```python
from build123d import *

# Parameters (mm, degrees)
SKETCH1_R                 = 10
BOSS_EXTRUDE1_DEPTH       = 25
FILLET2_R                 = 5
FILLET3_R                 = 5
F_3_0MM_DOWEL_HOLE1_D     = 3
F_3_0MM_DOWEL_HOLE1_DEPTH = 12.4
F_3_0MM_DOWEL_HOLE1_TIP   = 0.901290929


with BuildPart() as part:
    # Sketch1 → Boss-Extrude1 (new body)
    with BuildSketch(Plane(origin=(0, 0, 0), x_dir=(1, 0, 0), z_dir=(0, 1, 0))):
        with BuildLine():
            Line((0, 0), (-28, 0))
            Line((-28, 0), (-28, 8))
            Line((-28, 8), (-11.761010247, 8))
            ThreePointArc((-11.761010247, 8), (0, 32.310136302), (11.761010247, 8))
            Line((11.761010247, 8), (28, 8))
            Line((28, 8), (28, 0))
            Line((28, 0), (0, 0))
        make_face()
        with Locations(Location((0, 17.310136302, 0), (0, 0, 270))):
            Circle(SKETCH1_R, mode=Mode.SUBTRACT)
    extrude(amount=BOSS_EXTRUDE1_DEPTH)

    # Fillet2
    fillet2_edges = [part.edges().sort_by_distance(p)[0] for p in [
        (11.761010247, 12.5, -8),
    ]]
    fillet(fillet2_edges, radius=FILLET2_R)

    # Fillet3
    fillet3_edges = [part.edges().sort_by_distance(p)[0] for p in [
        (-11.761010247, 12.5, -8),
    ]]
    fillet(fillet3_edges, radius=FILLET3_R)

    # Ø3.0mm Dowel Hole1
    with Locations(Plane(origin=(23, 12.5, -8), x_dir=(-1, 0, 0), z_dir=(0, 0, -1))):
        with Locations((0, 0), (46.765023362, 0)):
            Hole(F_3_0MM_DOWEL_HOLE1_D / 2, depth=F_3_0MM_DOWEL_HOLE1_DEPTH)
            with Locations((0, 0, -(F_3_0MM_DOWEL_HOLE1_DEPTH + F_3_0MM_DOWEL_HOLE1_TIP / 2))):  # 118° drill point
                Cone(0, F_3_0MM_DOWEL_HOLE1_D / 2, F_3_0MM_DOWEL_HOLE1_TIP, mode=Mode.SUBTRACT)


solid = part.part
```
Geometry check sheet. Reference: the model listing, model coordinates, mm. A direction names the side the tool comes from. Give positions to 0.01 mm unless a question says otherwise; leave off trailing zeros. Order: outer loops, then holes, each group sorted by start corner. A loop starts at its lowest first (then second) coordinate and runs counter-clockwise, first axis right, second up. Notation, with made-up numbers: (1, 62) - (17, 62) arc R6 ccw to (17, 72) - close; hole circle Ø10 at (60, 85). An arc over 180 degrees is marked (long way). Answer in a Markdown table with one row per item. Add a question column.
Q1. Material ranges on probe 1 along Y at (x, z) = (23, -1); probe 2 along X at (y, z) = (4.25, -13.5); probe 3 along Z at (x, y) = (-24, 4.5), recorded low to high. Write a range as from..to.
Q2. Cross-section at A-A, the plane y = 12.5. Enter the section's corners in (x, z).
Q3. Gauge pin test, flat ends, axial feed: pin 1 (2.5 mm diameter, centred on x = -23.77, y = 12.5, fed in from +Z); pin 2 (8 mm diameter, centred on y = 5, z = -25, fed in from +X); pin 3 (4 mm diameter, centred on x = 23, y = 12.5, fed in from -Z); pin 4 (6 mm diameter, centred on y = 5.5, z = -20, fed in from +X). Record the tip position at first contact, or that the pin passes through.
Q4. Cross-section at B-B, the plane x = 23. Enter the section's corners in (y, z), then the cut area to 3 significant figures.
Q5. Mould release check, pull along X, two halves, no side actions. Record for faces 3 (the flat face through (25, 12, -8)), 4 (the flat face through (28, 12, -4)), 5 (the cylindrical face through (21.5, 12.57, -3.94)): pulls with the +X half, pulls with the -X half, needs draft (parallel to the pull), parting line crosses it, or undercut.
Q6. Cross-section at C-C, the plane z = -11.5. Enter the section's corners in (x, y), then the cut area to 3 significant figures.
Q7. Cross-section at D-D, the plane y = 4.5. Enter the section's corners in (x, z).
Q8. Tool access check on faces 1 (the flat face through (-22, 12, -8)), 2 (the flat face through (0, 0, -6)). Record the directions out of +Z, -Z, +X, -X, +Y, -Y that give a thin tool (end or side, any length) a straight path to the whole face; none if there is none.
Check values:
| question | item | result |
|---|---|---|
| 1 | probe 1 | y = 0..11, 14..25 |
| 1 | probe 2 | x = -14.56..-9.25, 9.25..14.56 |
| 1 | probe 3 | z = -8..0 |
| 2 | outline | (-28, -8) - (-25.27, -8) - (-25.27, 0) - (-28, 0) - close; (-22.27, -8) - (-19.53, -8) arc R5 cw to (-14.65, -14.08) arc R15 ccw (long way) to (14.65, -14.08) arc R5 cw to (19.53, -8) - (21.5, -8) - (21.5, 0) - (-22.27, 0) - close; (24.5, -8) - (28, -8) - (28, 0) - (24.5, 0) - close; hole circle Ø20 at (0, -17.31) |
| 3 | pin 1 | passes through |
| 3 | pin 2 | stops at x = 14.54 |
| 3 | pin 3 | stops at z = -8 |
| 3 | pin 4 | stops at x = 15 |
| 4 | outline | (0, -8) - (11, -8) - (11, 0) - (0, 0) - close; (14, -8) - (25, -8) - (25, 0) - (14, 0) - close |
| 4 | area | 176 mm^2 |
| 5 | face 3 | needs draft |
| 5 | face 4 | pulls with the +X half |
| 5 | face 5 | undercut |
| 6 | outline | (-14.76, 0) - (-8.14, 0) - (-8.14, 25) - (-14.76, 25) - close; (8.14, 0) - (14.76, 0) - (14.76, 25) - (8.14, 25) - close |
| 6 | area | 331 mm^2 |
| 7 | outline | (-28, -8) - (-19.53, -8) arc R5 cw to (-14.65, -14.08) arc R15 ccw (long way) to (14.65, -14.08) arc R5 cw to (19.53, -8) - (28, -8) - (28, 0) - (-28, 0) - close; hole circle Ø20 at (0, -17.31) |
| 8 | face 1 | -Z, -X, +Y, -Y |
| 8 | face 2 | +Z, -Z, +X, -X, -Y |
